Part model, mm, in its own coordinate system. A direction names the side the tool comes from. Give positions to 0.01 mm unless a question says otherwise; leave off trailing zeros. Write each loop counter-clockwise with the first axis right and the second up, starting at its lowest first coordinate (ties: lowest second). Pieces come first, ordered by that corner, then holes.
from build123d import *

# Parameters (mm, degrees)
SKETCH_1_W      = 29.3
SKETCH_1_H      = 5.45
EXTRUDE_1_DEPTH = 6
SKETCH_2_R      = 48.989794856
EXTRUDE_2_DEPTH = 100
SKETCH_3_R      = 50
EXTRUDE_3_DEPTH = 240


with BuildPart() as part:
    # Эскиз1 → Бобышка-Вытянуть1 (new body)
    with BuildSketch(Plane.XY):
        Polygon((0, 0), (-250, 0), (-250, -30), (-244.55, -30), (-244.55, -59.3), (-250, -59.3), (-250, -140.7), (-244.55, -140.7), (-244.55, -170), (-250, -170), (-250, -200), (-234.3, -200), (-234.3, -194.55), (-205, -194.55), (-205, -260), (-165, -329.282032303), (-85, -329.282032303), (-45, -260), (-45, -194.55), (-15.7, -194.55), (-15.7, -200), (0, -200), (0, -170), (-5.45, -170), (-5.45, -140.7), (0, -140.7), (0, -59.3), (-5.45, -59.3), (-5.45, -30), (0, -30), align=None)
        with Locations((-55, -128.825)):
            Rectangle(SKETCH_1_W, SKETCH_1_H, mode=Mode.SUBTRACT)
        with Locations((-195, -128.825)):
            Rectangle(SKETCH_1_W, SKETCH_1_H, mode=Mode.SUBTRACT)
        with Locations((-125, -128.825)):
            Rectangle(SKETCH_1_W, SKETCH_1_H, mode=Mode.SUBTRACT)
    extrude(amount=EXTRUDE_1_DEPTH)

    # Эскиз2 → Бобышка-Вытянуть2 (add)
    with BuildSketch(Plane.XY.offset(6)):
        with Locations(Location((-125, -260, 0), (0, 0, 180))):
            Circle(SKETCH_2_R)
    extrude(amount=EXTRUDE_2_DEPTH)

    # Эскиз3 → Бобышка-Вытянуть3 (add)
    with BuildSketch(Plane.XY.offset(6)):
        with Locations(Location((-185, -65, 0), (0, 0, 180))):
            Circle(SKETCH_3_R)
        with Locations(Location((-65, -65, 0), (0, 0, 180))):
            Circle(SKETCH_3_R)
    extrude(amount=EXTRUDE_3_DEPTH)


solid = part.part
1) Drill centre lines: L1, parallel to Z at x = -104.5, y = -202; L2, parallel to X at y = -261, z = 87.5; L3, parallel to Z at x = -91, y = -257.5. Where is each one in solid material? Low to high.
Check result:
L1: z = 0 to 6
L2: x = -173.98 to -76.02
L3: z = 0 to 106
2) Saw through at C-C (z = 100). Write the cut outline in (x, y), and give its area (3 significant figures).
Check result:
outline: circle Ø100 at (-185, -65); circle Ø97.98 at (-125, -260); circle Ø100 at (-65, -65)
area: 23,200 mm2
3) Mould opens along X. For faces 4 (the cylindrical face through (-86.123, -230.19, 55.3)), 5 (the cylindrical face through (-25, -35, 124)), 6 (the cylindrical face through (-135.05, -67.2, 124.32)), 7 (the flat face through (-126.7, -125.7, 0)) say: +X half, -X half, draft (parallel to the pull), parting line (faces both ways), or undercut.
Check result:
face 4: parting line
face 5: undercut
face 6: undercut
face 7: draft
4) Saw through at B-B (y = -65). Write the cut outline in (x, z).
Check result:
outline: (-250, 0) - (0, 0) - (0, 6) - (-15, 6) - (-15, 246) - (-115, 246) - (-115, 6) - (-135, 6) - (-135, 246) - (-235, 246) - (-235, 6) - (-250, 6) - close
5) Saw through at D-D (z = 215). Write the cut outline in (x, y).
Check result:
outline: circle Ø100 at (-185, -65); circle Ø100 at (-65, -65)
6) Flat gauge pins, fed straight in: P1, Ø6.5, axis at x = -62.5, z = 2, coming from the -Y side; P2, Ø5, axis at y = -84.5, z = 159, coming from the -X side; P3, Ø1.8, axis at y = -47.5, z = 2.5, coming from the +X side; P4, Ø2.5, axis at y = -129.5, z = 2.5, coming from the +X side. Where does each tip first touch, or does it go through?
Check result:
P1: stops at y = -295.94
P2: stops at x = -232.02
P3: stops at x = -5.45
P4: stops at x = 0
7) 3-axis set-ups, long thin cutter, end or side, ignore diameter. For faces 1 (the flat face through (-124, -261, 106)), 2 (the flat face through (-126.7, -125.7, 6)), 3 (the flat face through (-64, -66, 246)): which of +Z, -Z, +X, -X, +Y, -Y reach the whole face in a straight line?
Check result:
face 1: +Z, +X, -X, -Y
face 2: +Z
face 3: +Z, +X, -X, +Y, -Y
8) Saw through at A-A (x = -125). Write the cut outline in (y, z).
Check result:
outline: (-329.28, 0) - (-131.55, 0) - (-131.55, 6) - (-211.01, 6) - (-211.01, 106) - (-308.99, 106) - (-308.99, 6) - (-329.28, 6) - close; (-126.1, 0) - (0, 0) - (0, 6) - (-126.1, 6) - close
